Autodesk Inventor part; units mm, degrees
ref_plane "Work Plane1" through (2, 0, 0) normal (0, 0, 1) x (1, 0, 0)
ref_plane "YZ Plane" through (0, 0, 0) normal (1, 0, 0) x (0, 1, 0)
ref_plane "XZ Plane" through (0, 0, 0) normal (0, 1, 0) x (-1, 0, 0)
sketch "Sketch1" plane through (0, 0, 0) normal (0, 1, 0) x (-1, 0, 0)
  line L0 (-2, -25) -> (-50, -25)
  line L1 (-50, -25) -> (-50, 0)
  line L2 (-2, 0) -> (-2, -25)
  line L3 (0, 0) -> (-2, 0)
  line L4 (-46, 0) -> (-50, 0)
  line L5 (-6, -17) -> (-46, -17)
  line L6 (-46, -17) -> (-46, 0)
  line L7 (-6, 0) -> (-6, -17)
  line L8 (-2, 0) -> (-6, 0)
  line L9 (-50, 0) -> (-46, 0)
  line L10 (-2, 0) -> (0, 0)
  dimension "d3" = 48
  dimension "d4" = 40
  dimension "d7" = 4
  dimension "d8" = 4
  dimension "d10" = 25
  dimension "d12" = 17
extrude "Extrusion1" add sketch "Sketch1" along normal blind 4
sketch "Sketch2" plane through (0, 0, 0) normal (0, -1, 0) x (1, 0, 0)
  circle A0 centre (6, -29) radius 2.1
  arc A1 (2, -29) -> (10, -29) centre (6, -29) ccw
  line L0 (50, -25) -> (2, -25)
  line L1 (2, -25) -> (2, 0)
  line L2 (2, -25) -> (2, -29)
  line L3 (10, -29) -> (10, -25)
  circle A2 centre (46, -29) radius 2.1
  arc A3 (42, -29) -> (50, -29) centre (46, -29) ccw
  line L4 (50, 0) -> (50, -25)
  line L5 (50, -25) -> (50, -29)
  line L6 (42, -29) -> (42, -25)
  point P0 (0, 0)
  dimension "d13" = 4.2
  dimension "d14" = 8
  dimension "d15" = 4
  dimension "d16" = 4
  dimension "d17" = 4.2
  dimension "d18" = 8
  dimension "d19" = 4
  dimension "d20" = 4
extrude "Extrusion2" add sketch "Sketch2" against normal blind 2
ref_plane "Work Plane1" through (2, 0, 0) normal (0, 0, 1) x (1, 0, 0)
sketch "Sketch3" plane through (2, 0, 0) normal (0, 0, 1) x (1, 0, 0)
  line L0 (0, 0) -> (4, 0)
  line L1 (4, 0) -> (4, 4)
  line L2 (0, 4) -> (4, 4)
  line L3 (0, 0) -> (0, 4)
  line L4 (44, 0) -> (48, 0)
  line L5 (48, 0) -> (48, 4)
  line L6 (44, 4) -> (48, 4)
  line L7 (44, 0) -> (44, 4)
  line L8 (1, 3) -> (4, 3)
  line L9 (4, 3) -> (4, 1)
  line L10 (4, 1) -> (1, 1)
  line L11 (1, 1) -> (1, 3)
  line L12 (44, 3) -> (47, 3)
  line L13 (47, 3) -> (47, 1)
  line L14 (47, 1) -> (44, 1)
  line L15 (44, 1) -> (44, 3)
  point P0 (-2, 0)
  dimension "d24" = 3
  dimension "d25" = 2
  dimension "d26" = 1
  dimension "d27" = 0
  dimension "d28" = 3
  dimension "d29" = 2
  dimension "d30" = 1
  dimension "d31" = 0
extrude "Extrusion3" cut sketch "Sketch3" against normal up to surface (17 mm away) contours L10 L11 L8 L1 | L7 L12 L13 L14
properties part number "Electronics-Wedge-small"
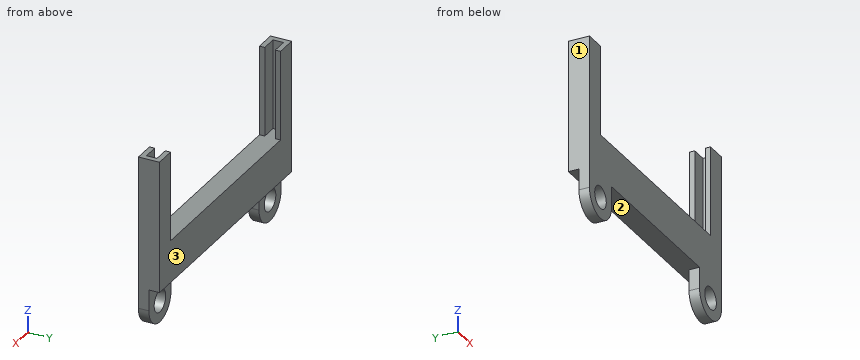
The model under review builds one solid part; all positions refer to its coordinate system, in mm. Face numbers are marked on the shaded views. Give positions to 0.01 mm unless a question says otherwise; leave off trailing zeros. Loops run counter-clockwise (first coordinate to the right, second up) from the corner with the lowest first, then second, coordinate; pieces in that order, holes last. Notation, with made-up numbers: (40, 88.5) - (53, 88.5) arc R13 ccw to (53, 99.5) - close; hole circle Ø11 at (56, 37). An arc over 180 degrees is marked (long way). Answer as a JSON object with one key per item and string values.
Q1. Mouldability with a two-part tool opening along X and no side actions: class the marked faces 1, 2 and 3 as +X half, -X half, draft (parallel to the pull), parting line (faces both ways), or undercut.
Worked out:
{"face 1": "-X half", "face 2": "undercut", "face 3": "draft"}
Q2. Add section C-C on z = -28.5. State the section outline as (x, y) points.
Worked out:
{"outline": "(2, 0) - (3.96, 0) - (3.96, 2) - (2, 2) - close; (8.04, 0) - (10, 0) - (10, 2) - (8.04, 2) - close; (42, 0) - (43.96, 0) - (43.96, 2) - (42, 2) - close; (48.04, 0) - (50, 0) - (50, 2) - (48.04, 2) - close"}
Q3. Insertion check: pin 1 (9 mm diameter, centred on x = 44.5, z = -30, fed in from +Y); pin 2 (2 mm diameter, centred on x = 21.5, y = 1, fed in from -Z). Each pin has a flat end and moves straight along its axis. Give the tip position at first contact, or say it passes through.
Worked out:
{"pin 1": "stops at y = 2", "pin 2": "stops at z = -25"}
Q4. Add section B-B on y = 3.5. State the section outline as (x, z) points, plus the area to 3 significant figures.
Worked out:
{"outline": "(2, -25) - (50, -25) - (50, 0) - (46, 0) - (46, -17) - (6, -17) - (6, 0) - (2, 0) - close", "area": "520 mm^2"}
Q5. Add section A-A on z = -1.5. State the section outline as (x, y) points, plus the area to 3 significant figures.
Worked out:
{"outline": "(2, 0) - (6, 0) - (6, 1) - (3, 1) - (3, 3) - (6, 3) - (6, 4) - (2, 4) - close; (46, 0) - (50, 0) - (50, 4) - (46, 4) - (46, 3) - (49, 3) - (49, 1) - (46, 1) - close", "area": "20.0 mm^2"}
Q6. Add section D-D on x = 23.5. State the section outline as (y, z) points, plus the area to 3 significant figures.
Worked out:
{"outline": "(0, -25) - (4, -25) - (4, -17) - (0, -17) - close", "area": "32.0 mm^2"}
Q7. To check wall thickness, follow line 1 along Z through (x, y) = (6, 1.4); line 2 along X through (y, z) = (3.8, -14.5); line 3 along X through (y, z) = (1.1, -2). State the ranges of each line that lie inside material, in increasing order.
Worked out:
{"line 1": "z = -33 to -31.1, -26.9 to -17", "line 2": "x = 2 to 6, 46 to 50", "line 3": "x = 2 to 3, 49 to 50"}
